```python
from build123d import *

# Parameters (mm, degrees)
SKETCH1_W           = 57.15
SKETCH1_H           = 25.4
BOSS_EXTRUDE1_DEPTH = 43.65625
FILLET1_R           = 3.175
CUT_EXTRUDE1_DEPTH  = 0.79375
SKETCH3_R           = 1.984375
CUT_EXTRUDE2_DEPTH  = 0.79375
BOSS_EXTRUDE2_DEPTH = 2.38125
CHAMFER1_SIZE       = 2.38125
SKETCH5_R           = 2.778125
SKETCH5_R_2         = 3.571875
BOSS_EXTRUDE3_DEPTH = 2.38125
CHAMFER2_SIZE       = 0.79375
SKETCH6_R           = 3.683
SKETCH6_R_2         = 2.286
BOSS_EXTRUDE4_DEPTH = 3.175
SKETCH7_R           = 5.461
BOSS_EXTRUDE5_DEPTH = 3.429
SKETCH8_R           = 1.27
BOSS_EXTRUDE6_DEPTH = 3.175
SKETCH9_R           = 1.905
BOSS_EXTRUDE7_DEPTH = 25.4
FILLET2_R           = 1.27
CUT_EXTRUDE3_START  = -1.5875
SKETCH10_R          = 5.461
SKETCH10_R_2        = 3.96875
CUT_EXTRUDE3_DEPTH  = 1.5875


# Some blends are built 0.0001 mm under size
with BuildPart() as part:
    # Sketch1 → Boss-Extrude1 (new body)
    with BuildSketch(Plane(origin=(0, 0, 0), x_dir=(1, 0, 0), z_dir=(0, 1, 0))):
        Rectangle(SKETCH1_W, SKETCH1_H)
    extrude(amount=BOSS_EXTRUDE1_DEPTH)

    # Fillet1
    fillet1_edges = [part.edges().sort_by_distance(p)[0] for p in [
        (28.575, 21.828125, 12.7),
        (-28.575, 21.828125, 12.7),
        (-28.575, 21.828125, -12.7),
        (28.575, 21.828125, -12.7),
    ]]
    fillet(fillet1_edges, radius=FILLET1_R)

    # Sketch2 → Cut-Extrude1 (cut)
    with BuildSketch(Plane(origin=(0, 43.65625, 0), x_dir=(1, 0, 0), z_dir=(0, 1, 0))):
        with BuildLine():
            Line((25.4, 11.8745), (-25.4, 11.8745))
            ThreePointArc((-25.4, 11.8745), (-27.061347382, 11.186347382), (-27.7495, 9.525))
            Line((-27.7495, 9.525), (-27.7495, -9.525))
            ThreePointArc((-27.7495, -9.525), (-27.061347382, -11.186347382), (-25.4, -11.8745))
            Line((-25.4, -11.8745), (25.4, -11.8745))
            ThreePointArc((25.4, -11.8745), (27.061347382, -11.186347382), (27.7495, -9.525))
            Line((27.7495, -9.525), (27.7495, 9.525))
            ThreePointArc((27.7495, 9.525), (27.061347382, 11.186347382), (25.4, 11.8745))
        make_face()
        with BuildLine():
            Line((25.4, 11.176), (-25.4, 11.176))
            ThreePointArc((-25.4, 11.176), (-26.567433296, 10.692433296), (-27.051, 9.525))
            Line((-27.051, 9.525), (-27.051, -9.525))
            ThreePointArc((-27.051, -9.525), (-26.567433296, -10.692433296), (-25.4, -11.176))
            Line((-25.4, -11.176), (25.4, -11.176))
            ThreePointArc((25.4, -11.176), (26.567433296, -10.692433296), (27.051, -9.525))
            Line((27.051, -9.525), (27.051, 9.525))
            ThreePointArc((27.051, 9.525), (26.567433296, 10.692433296), (25.4, 11.176))
        make_face(mode=Mode.SUBTRACT)
    extrude(amount=-CUT_EXTRUDE1_DEPTH, mode=Mode.SUBTRACT)

    # Sketch3 → Cut-Extrude2 (cut)
    with BuildSketch(Plane(origin=(0, 43.65625, 0), x_dir=(1, 0, 0), z_dir=(0, 1, 0))):
        with Locations(Location((-23.8125, 8.73125, 0), (0, 0, 270))):
            Circle(SKETCH3_R)
        with Locations(Location((-23.8125, -8.73125, 0), (0, 0, 270))):
            Circle(SKETCH3_R)
        with Locations(Location((23.8125, -8.73125, 0), (0, 0, 270))):
            Circle(SKETCH3_R)
        with Locations(Location((23.8125, 8.73125, 0), (0, 0, 270))):
            Circle(SKETCH3_R)
    extrude(amount=-CUT_EXTRUDE2_DEPTH, mode=Mode.SUBTRACT)

    # Sketch4 → Boss-Extrude2 (add)
    with BuildSketch(Plane(origin=(0, 43.65625, 0), x_dir=(1, 0, 0), z_dir=(0, 1, 0))):
        with BuildLine():
            Line((22.492963736, -11.176), (-22.492963736, -11.176))
            ThreePointArc((-22.492963736, -11.176), (-21.446391914, -7.275395941), (-25.4, -6.4513767))
            Line((-25.4, -6.4513767), (-25.4, 6.4513767))
            ThreePointArc((-25.4, 6.4513767), (-21.446391914, 7.275395941), (-22.492963736, 11.176))
            Line((-22.492963736, 11.176), (22.492963736, 11.176))
            ThreePointArc((22.492963736, 11.176), (21.446391914, 7.275395941), (25.4, 6.4513767))
            Line((25.4, 6.4513767), (25.4, -6.4513767))
            ThreePointArc((25.4, -6.4513767), (21.446391914, -7.275395941), (22.492963736, -11.176))
        make_face()
    extrude(amount=BOSS_EXTRUDE2_DEPTH)

    # Chamfer1
    chamfer1_edges = [part.edges().sort_by_distance(p)[0] for p in [
        (25.4, 46.0375, 0),
        (0, 46.0375, -11.176),
        (-25.4, 46.0375, 0),
        (0, 46.0375, 11.176),
    ]]
    chamfer(chamfer1_edges, length=CHAMFER1_SIZE - 0.0001)  # a hair under: the kernel refuses the full size

    # Sketch5 → Boss-Extrude3 (add)
    with BuildSketch(Plane(origin=(0, 46.0375, 0), x_dir=(1, 0, 0), z_dir=(0, 1, 0))):
        with Locations((1.905, 7.14375)):
            Circle(SKETCH5_R)
        with Locations((1.905, -7.14375)):
            Circle(SKETCH5_R)
        with Locations((-22.51075, 0)):
            Circle(SKETCH5_R_2)
    extrude(amount=-BOSS_EXTRUDE3_DEPTH)

    # Chamfer2
    chamfer2_edges = [part.edges().sort_by_distance(p)[0] for p in [
        (-26.082625, 46.0375, 0),
    ]]
    chamfer(chamfer2_edges, length=CHAMFER2_SIZE)

    # Sketch6 → Boss-Extrude4 (add)
    # profile 1 of 2: a face of its own
    with BuildSketch(Plane(origin=(0, 46.0375, 0), x_dir=(1, 0, 0), z_dir=(0, 1, 0))):
        with Locations(Location((3.15087, 0, 0), (0, 0, 270))):
            Circle(SKETCH6_R)
        with Locations(Location((3.15087, 0, 0), (0, 0, 270))):
            Circle(SKETCH6_R_2, mode=Mode.SUBTRACT)
    # profile 2 of 2: a face of its own
    with BuildSketch(Plane(origin=(0, 46.0375, 0), x_dir=(1, 0, 0), z_dir=(0, 1, 0))):
        with Locations(Location((15.85087, 0, 0), (0, 0, 270))):
            Circle(SKETCH6_R)
        with Locations(Location((15.85087, 0, 0), (0, 0, 270))):
            Circle(SKETCH6_R_2, mode=Mode.SUBTRACT)
    extrude(amount=BOSS_EXTRUDE4_DEPTH)

    # Sketch7 → Boss-Extrude5 (add)
    with BuildSketch(Plane(origin=(0, 46.0375, 0), x_dir=(1, 0, 0), z_dir=(0, 1, 0))):
        with Locations(Location((-9.54913, 0, 0), (0, 0, 270))):
            Circle(SKETCH7_R)
    extrude(amount=BOSS_EXTRUDE5_DEPTH)

    # Sketch8 → Boss-Extrude6 (add)
    with BuildSketch(Plane(origin=(0, 42.8625, 0), x_dir=(1, 0, 0), z_dir=(0, 1, 0))):
        with Locations(Location((-23.8125, -8.73125, 0), (0, 0, 270))):
            Circle(SKETCH8_R)
        with Locations(Location((23.8125, -8.73125, 0), (0, 0, 270))):
            Circle(SKETCH8_R)
        with Locations(Location((23.8125, 8.73125, 0), (0, 0, 270))):
            Circle(SKETCH8_R)
        with Locations(Location((-23.8125, 8.73125, 0), (0, 0, 270))):
            Circle(SKETCH8_R)
    extrude(amount=BOSS_EXTRUDE6_DEPTH)

    # Sketch9 → Boss-Extrude7 (add)
    with BuildSketch(Plane(origin=(0, 46.0375, 0), x_dir=(1, 0, 0), z_dir=(0, 1, 0))):
        with Locations(Location((-23.8125, -8.73125, 0), (0, 0, 270))):
            Circle(SKETCH9_R)
        with Locations(Location((-23.8125, 8.73125, 0), (0, 0, 270))):
            Circle(SKETCH9_R)
        with Locations(Location((23.8125, 8.73125, 0), (0, 0, 270))):
            Circle(SKETCH9_R)
        with Locations(Location((23.8125, -8.73125, 0), (0, 0, 270))):
            Circle(SKETCH9_R)
    extrude(amount=BOSS_EXTRUDE7_DEPTH)

    # Fillet2
    # the kernel refuses this fillet: 1.27 mm, written as the material it takes off along each edge
    with BuildSketch(Plane(origin=(23.8125, 46.0375, 8.73125), x_dir=(0, 0, 1), z_dir=(-1, 0, 0))) as fillet2_piece_1:
        with BuildLine():
            CenterArc((0.635, 1.099852263), FILLET2_R, 300, 60)
            Line((1.905, 1.099852263), (1.9304, 1.099852263))
            Line((1.9304, 1.099852263), (1.9304, 0))
            Line((1.9304, 0), (1.905, -0.0254))
            ThreePointArc((1.905, -0.0254), (1.5875, -0.0254), (1.2827, -0.021997045))
            Line((1.2827, -0.021997045), (1.27, 0))
        make_face()
    revolve(axis=Axis((23.8125, 46.0375, 8.73125), (0, 1, 0)), mode=Mode.SUBTRACT)
    with BuildSketch(Plane(origin=(23.8125, 46.0375, -8.73125), x_dir=(0, 0, 1), z_dir=(-1, 0, 0))) as fillet2_piece_2:
        with BuildLine():
            CenterArc((0.635, 1.099852263), FILLET2_R, 300, 60)
            Line((1.905, 1.099852263), (1.9304, 1.099852263))
            Line((1.9304, 1.099852263), (1.9304, 0))
            Line((1.9304, 0), (1.905, -0.0254))
            ThreePointArc((1.905, -0.0254), (1.5875, -0.0254), (1.2827, -0.021997045))
            Line((1.2827, -0.021997045), (1.27, 0))
        make_face()
    revolve(axis=Axis((23.8125, 46.0375, -8.73125), (0, 1, 0)), mode=Mode.SUBTRACT)
    with BuildSketch(Plane(origin=(-23.8125, 46.0375, -8.73125), x_dir=(0, 0, 1), z_dir=(-1, 0, 0))) as fillet2_piece_3:
        with BuildLine():
            CenterArc((0.635, 1.099852263), FILLET2_R, 300, 60)
            Line((1.905, 1.099852263), (1.9304, 1.099852263))
            Line((1.9304, 1.099852263), (1.9304, 0))
            Line((1.9304, 0), (1.905, -0.0254))
            ThreePointArc((1.905, -0.0254), (1.5875, -0.0254), (1.2827, -0.021997045))
            Line((1.2827, -0.021997045), (1.27, 0))
        make_face()
    revolve(axis=Axis((-23.8125, 46.0375, -8.73125), (0, 1, 0)), mode=Mode.SUBTRACT)
    with BuildSketch(Plane(origin=(-23.8125, 46.0375, 8.73125), x_dir=(0, 0, 1), z_dir=(-1, 0, 0))) as fillet2_piece_4:
        with BuildLine():
            CenterArc((0.635, 1.099852263), FILLET2_R, 300, 60)
            Line((1.27, 0), (1.2827, -0.021997045))
            ThreePointArc((1.2827, -0.021997045), (1.5875, -0.0254), (1.905, -0.0254))
            Line((1.905, -0.0254), (1.9304, 0))
            Line((1.9304, 0), (1.9304, 1.099852263))
            Line((1.9304, 1.099852263), (1.905, 1.099852263))
        make_face()
    revolve(axis=Axis((-23.8125, 46.0375, 8.73125), (0, 1, 0)), mode=Mode.SUBTRACT)

    # Sketch10 → Cut-Extrude3 (cut)
    with BuildSketch(Plane(origin=(0, 49.4665, 0), x_dir=(1, 0, 0), z_dir=(0, 1, 0)).offset(CUT_EXTRUDE3_START)):
        with Locations(Location((-9.54913, 0, 0), (0, 0, 270))):
            Circle(SKETCH10_R)
        with Locations(Location((-9.54913, 0, 0), (0, 0, 270))):
            Circle(SKETCH10_R_2, mode=Mode.SUBTRACT)
    extrude(amount=CUT_EXTRUDE3_DEPTH, mode=Mode.SUBTRACT)


solid = part.part
```
The model under review builds one solid part; all positions refer to its coordinate system, in mm. A direction names the side the tool comes from. Coordinates: 2 decimals unless noted, no trailing zeros. Write each loop counter-clockwise with the first axis right and the second up, starting at its lowest first coordinate (ties: lowest second). Pieces come first, ordered by that corner, then holes. Notation, with made-up numbers: (35, -14.75) - (50, -14.75) arc R11 cw to (50, -4.75) - close; hole circle Ø9 at (-9, -32.5). An arc over 180 degrees is marked (long way). Answer in a Markdown table with one row per item. Add a question column.
Q1. Consider section A-A on x = -17. Give the boundary of the cut face in (y, z).
Q2. To check wall thickness, follow line 1 along X through (y, z) = (47.95, 0); line 2 along X through (y, z) = (47.2, 0); line 3 along X through (y, z) = (43, 0) (1 decimal). State the ranges of each line that lie inside material, in increasing order. Write a range as from..to.
Q3. Clearance check with flat-ended pins moving along their axes: pin 1 (5 mm diameter, centred on x = -21, z = -0.5, fed in from +Y); pin 2 (8 mm diameter, centred on x = 16.5, z = -0.5, fed in from +Y); pin 3 (10 mm diameter, centred on x = -20.5, y = 64.5, fed in from +Z). State where each tip first meets the part, or that it passes through.
Q4. Consider section D-D on x = 2. Give the boundary of the cut face in (y, z).
Q5. Consider section B-B on y = 59. Give the boundary of the cut face in (x, z) (1 decimal), then the cut area to 3 significant figures.
Q6. For faces 1 (the face through (-24, 71.438, 9)), 2 (the face through (3, 46.038, 0)), 3 (the face through (-24.226, 44.83, 4.306)), list the 3-axis set-ups (+Z, -Z, +X, -X, +Y, -Y) from which the entire face can be reached by the end or side of a thin tool; tool diameter is ignored.
Q7. Consider section C-C on x = -8. Give the boundary of the cut face in (y, z).
Q8. Draft analysis for pull direction Y (two halves, no side actions). For faces 4 (the face through (-24, 71.438, -9)), 5 (the face through (-24, 42.862, -7)), 6 (the face through (-25.672, 59.117, 8.318)), state which applies: +Y half, -Y half, draft (parallel to the pull), parting line (faces both ways), or undercut.
Answers below:
| question | item | result |
|---|---|---|
| 1 | outline | (0, -12.7) - (43.66, -12.7) - (43.66, -11.87) - (42.86, -11.87) - (42.86, -11.18) - (43.66, -11.18) - (46.04, -8.79) - (46.04, 8.79) - (43.66, 11.18) - (42.86, 11.18) - (42.86, 11.87) - (43.66, 11.87) - (43.66, 12.7) - (0, 12.7) - close |
| 2 | line 1 | -13.52..-5.58, -0.53..0.86, 5.44..6.83, 12.17..13.56, 18.14..19.53 |
| 2 | line 2 | -15.01..-4.09, -0.53..0.86, 5.44..6.83, 12.17..13.56, 18.14..19.53 |
| 2 | line 3 | -28.6..-27.7, -27.1..27.1, 27.7..28.6 |
| 3 | pin 1 | y = 46.04 |
| 3 | pin 2 | y = 49.21 |
| 3 | pin 3 | z = 10.64 |
| 4 | outline | (0, -12.7) - (43.66, -12.7) - (43.66, -11.87) - (42.86, -11.87) - (42.86, -11.18) - (43.66, -11.18) - (44.91, -9.92) - (46.04, -9.92) - (46.04, -3.5) - (49.21, -3.5) - (49.21, -1.98) - (46.04, -1.98) - (46.04, 1.98) - (49.21, 1.98) - (49.21, 3.5) - (46.04, 3.5) - (46.04, 9.92) - (44.91, 9.92) - (43.66, 11.18) - (42.86, 11.18) - (42.86, 11.87) - (43.66, 11.87) - (43.66, 12.7) - (0, 12.7) - close |
| 5 | outline | circle Ø3.8 at (-23.8, -8.7); circle Ø3.8 at (-23.8, 8.7); circle Ø3.8 at (23.8, -8.7); circle Ø3.8 at (23.8, 8.7) |
| 5 | area | 45.6 mm² |
| 6 | face 1 | +Z, -Z, +X, -X, +Y |
| 6 | face 2 | +Y |
| 6 | face 3 | -X, +Y |
| 7 | outline | (0, -12.7) - (43.66, -12.7) - (43.66, -11.87) - (42.86, -11.87) - (42.86, -11.18) - (43.66, -11.18) - (46.04, -8.79) - (46.04, -5.24) - (47.88, -5.24) - (47.88, -3.65) - (49.47, -3.65) - (49.47, 3.65) - (47.88, 3.65) - (47.88, 5.24) - (46.04, 5.24) - (46.04, 8.79) - (43.66, 11.18) - (42.86, 11.18) - (42.86, 11.87) - (43.66, 11.87) - (43.66, 12.7) - (0, 12.7) - close |
| 8 | face 4 | +Y half |
| 8 | face 5 | undercut |
| 8 | face 6 | draft |
